Read the model definition and answer for the solid it produces. Units are mm, in the model's axes. Coordinates: 2 decimals unless noted, no trailing zeros. Loops run counter-clockwise (first coordinate to the right, second up) from the corner with the lowest first, then second, coordinate; pieces in that order, holes last. Notation, with made-up numbers: (15.5, 37.25) - (46.5, 37.25) arc R26 ccw to (46.5, 71.25) - close; hole circle Ø10 at (17, 3.25). An arc over 180 degrees is marked (long way). Use one line per item in the form item = value.
from build123d import *

# Parameters (mm, degrees)
SKETCH1_R           = 28.35
SKETCH1_R_2         = 21.55
EXTRUDE_THIN1_DEPTH = 2
CHAMFER1_SIZE       = 0.5
SKETCH2_R           = 1.25
CUT_EXTRUDE1_DEPTH  = 41.142807575
CIRPATTERN1_COUNT   = 4
CHAMFER2_SIZE       = 0.25


with BuildPart() as part:
    # Sketch1 → Extrude-Thin1 (new body)
    with BuildSketch(Plane(origin=(0, 0, 0), x_dir=(0, 1, 0), z_dir=(0, 0, 1))):
        Circle(SKETCH1_R)
        Circle(SKETCH1_R_2, mode=Mode.SUBTRACT)
    extrude(amount=EXTRUDE_THIN1_DEPTH)

    # Chamfer1
    chamfer1_edges = [part.edges().sort_by_distance(p)[0] for p in [
        (0, -21.55, 0),
        (0, -21.55, 2),
    ]]
    chamfer(chamfer1_edges, length=CHAMFER1_SIZE)

    # Sketch2 → Cut-Extrude1 (cut, through all)
    with BuildSketch(Plane(origin=(0, 0, 0), x_dir=(0, 1, 0), z_dir=(0, 0, 1))):
        with Locations(Location((0, 26.3, 0), (0, 0, 270))):
            Circle(SKETCH2_R)
    cut_extrude1 = extrude(amount=CUT_EXTRUDE1_DEPTH, mode=Mode.SUBTRACT)

    # CirPattern1: Cut-Extrude1 ×4 about axis
    cirpattern1_axis = Axis((0, 0, 0), (0, 0, 1))
    for i in range(1, CIRPATTERN1_COUNT):
        add(cut_extrude1.rotate(cirpattern1_axis, i * 360 / CIRPATTERN1_COUNT), mode=Mode.SUBTRACT)

    # Chamfer2
    chamfer2_edges = [part.edges().sort_by_distance(p)[0] for p in [
        (-27.55, 0, 0),
        (-27.55, 0, 2),
        (0, 27.55, 0),
        (0, 27.55, 2),
        (27.55, 0, 0),
        (27.55, 0, 2),
        (0, -27.55, 0),
        (0, -27.55, 2),
    ]]
    chamfer(chamfer2_edges, length=CHAMFER2_SIZE)


solid = part.part
Item 1: Find the intervals of material crossed by L1, parallel to X at y = 0, z = 0.7; L2, parallel to X at y = -3, z = 1.1; L3, parallel to X at y = 6.5, z = 1.75, in increasing order.
Results below:
L1 = -28.35 to -27.55, -25.05 to -21.55, 21.55 to 25.05, 27.55 to 28.35
L2 = -28.19 to -21.34, 21.34 to 28.19
L3 = -27.59 to -20.81, 20.81 to 27.59
Item 2: The part is cut by section B-B on z = 0.9. Give the vertices of the cut face in (x, y), plus the area to 3 significant figures.
Results below:
outline = circle Ø56.7 at (0, 0); hole circle Ø2.5 at (-26.3, 0); hole circle Ø43.1 at (0, 0); hole circle Ø2.5 at (0, -26.3); hole circle Ø2.5 at (0, 26.3); hole circle Ø2.5 at (26.3, 0)
area = 1,050 mm²
Item 3: The part is cut by section C-C on y = -26.3. Give the vertices of the cut face in (x, z).
Results below:
outline = (-10.58, 0) - (-1.5, 0) - (-1.25, 0.25) - (-1.25, 1.75) - (-1.5, 2) - (-10.58, 2) - close; (1.25, 0.25) - (1.5, 0) - (10.58, 0) - (10.58, 2) - (1.5, 2) - (1.25, 1.75) - close
Item 4: This flat-tipped pin is pushed along its axis until it touches: P1, Ø1, axis at x = -1.5, z = 1.5, coming from the -Y side. Where does it stop, or does it pass through?
Results below:
P1 = -28.33
Item 5: The part is cut by section A-A on x = 0. Give the vertices of the cut face in (y, z).
Results below:
outline = (-28.35, 0) - (-27.8, 0) - (-27.55, 0.25) - (-27.55, 1.75) - (-27.8, 2) - (-28.35, 2) - close; (-25.05, 0.25) - (-24.8, 0) - (-22.05, 0) - (-21.55, 0.5) - (-21.55, 1.5) - (-22.05, 2) - (-24.8, 2) - (-25.05, 1.75) - close; (21.55, 0.5) - (22.05, 0) - (24.8, 0) - (25.05, 0.25) - (25.05, 1.75) - (24.8, 2) - (22.05, 2) - (21.55, 1.5) - close; (27.55, 0.25) - (27.8, 0) - (28.35, 0) - (28.35, 2) - (27.8, 2) - (27.55, 1.75) - close
Item 6: For a pull along Y with two mould halves and no side action, classify faces 1 (the flat face through (-17, 15, 0)), 2 (the cylindrical face through (-23.905, 15.241, 0.986)), 3 (the cylindrical face through (-0.479, 25.145, 0.99)) as +Y half, -Y half, draft (parallel to the pull), parting line (faces both ways), or undercut.
Results below:
face_1 = draft
face_2 = parting line
face_3 = undercut
